For this review, take the finished solid that the model builds, in its own axes (mm). A direction names the side the tool comes from. Coordinates: 2 decimals unless noted, no trailing zeros. Loops run counter-clockwise (first coordinate to the right, second up) from the corner with the lowest first, then second, coordinate; pieces in that order, holes last. Notation, with made-up numbers: (39, -32) - (49, -32) arc R9 cw to (49, -28) - close; hole circle Ø10 at (67.5, -19.5). An arc over 180 degrees is marked (long way). One line per item, written item: value. Start each with the question number.
1. Take a section at C-C, the plane x = 0. Count the separate pieces of the cut face and the enclosed holes in it, and give its area (3 significant figures).
2. To check wall thickness, follow line 1 (X direction, y = 19, z = 0.5); line 2 (X direction, y = 16.75, z = -7); line 3 (Y direction, x = -2.25, z = -12.5). State the ranges of each line that lie inside material, in increasing order. Write a range as from..to.
3. Take a section at B-B, the plane y = 18.25. State the section outline as (x, z) points, and give its area (3 significant figures).
4. Take a section at A-A, the plane x = 3.75. State the section outline as (y, z) points, and give its area (4 significant figures).
5. For faces 1 (the face through (-0.05, 21.48, 1.48)), 2 (the face through (-8, 21, -8)), 3 (the face through (-5, 31, 0)), 4 (the face through (0, 5.98, 3)), list the 3-axis set-ups (+Z, -Z, +X, -X, +Y, -Y) from which the entire face can be reached by the end or side of a thin tool; tool diameter is ignored.
6. The part is to be moulded in two halves that separate along X. For faces 5 (the face through (8.986, 15.805, -12.325)), 6 (the face through (-2.15, 18, 1)), 7 (the face through (10, 22, -6)), say which applies: released by +X, released by -X, zero draft, split by the parting line, or undercut.
7. Insertion check: pin 1 (8 mm diameter, centred on x = 6, z = -17, fed in from +Y); pin 2 (0.9 mm diameter, centred on x = -1.5, y = 6.5, fed in from +Z); pin 3 (6 mm diameter, centred on x = -7.5, y = 23.5, fed in from -Z). Each pin has a flat end and moves straight along its axis. Give the tip position at first contact, or say it passes through.
8. Take a section at D-D, the plane y = 14. State the section outline as (x, z) points.
```python
from build123d import *

# Parameters (mm, degrees)
SKETCH_1_W               = 20
SKETCH_1_H               = 28
EXTRUDE_1_DEPTH          = 3
SKETCH_2_W               = 10
SKETCH_2_H               = 3
CUT_EXTRUDE_1_DEPTH      = 1
SKETCH_3_W               = 4
SKETCH_3_H               = 1
EXTRUDE_2_DEPTH          = 1.5
MIRROR_2_COPY_1_SKETCH_W = 10
MIRROR_2_COPY_1_SKETCH_H = 3
MIRROR_2_COPY_1_DEPTH    = 1
MIRROR_2_COPY_2_SKETCH_W = 4
MIRROR_2_COPY_2_SKETCH_H = 1
MIRROR_2_COPY_2_DEPTH    = 1.5
RIB_2_REACH              = 47.252
SKETCH_4_WALL_W          = 127.859233498
SKETCH_4_WALL_H          = 2


with BuildPart() as part:
    # 草图1 → 凸台-拉伸1 (new body)
    with BuildSketch(Plane.XY):
        with Locations((0, 17.480286539)):
            Rectangle(SKETCH_1_W, SKETCH_1_H)
        with BuildLine():
            Line((2.15, 19.330286539), (2.15, 16.830286539))
            ThreePointArc((2.15, 16.830286539), (0, 14.680286539), (-2.15, 16.830286539))
            Line((-2.15, 16.830286539), (-2.15, 19.330286539))
            ThreePointArc((-2.15, 19.330286539), (0, 21.480286539), (2.15, 19.330286539))
        make_face(mode=Mode.SUBTRACT)
    extrude_1 = extrude(amount=EXTRUDE_1_DEPTH)

    # 草图2 → 切除-拉伸1 (cut)
    with BuildSketch(Plane.XY.offset(3)):
        with Locations((0, 28.480286539)):
            Rectangle(SKETCH_2_W, SKETCH_2_H)
    cut_extrude_1 = extrude(amount=-CUT_EXTRUDE_1_DEPTH, mode=Mode.SUBTRACT)

    # 草图3 → 凸台-拉伸2 (add)
    with BuildSketch(Plane.XY.offset(2)):
        with Locations((0, 29.480286539)):
            Rectangle(SKETCH_3_W, SKETCH_3_H)
    extrude_2 = extrude(amount=EXTRUDE_2_DEPTH)

    # 镜向1: 切除-拉伸1, 凸台-拉伸2 across plane
    add(cut_extrude_1.mirror(Plane.ZX.offset(17.480286539)), mode=Mode.SUBTRACT)
    add(extrude_2.mirror(Plane.ZX.offset(17.480286539)))

    # 镜向2: 凸台-拉伸1, 切除-拉伸1, 凸台-拉伸2 across plane
    add(extrude_1.mirror(Plane(origin=(0, 14.240143269, -14.240143269), x_dir=(0, 0.7071067811865478, 0.7071067811865472), z_dir=(0, -0.7071067811865475, 0.7071067811865477))))
    add(cut_extrude_1.mirror(Plane(origin=(0, 14.240143269, -14.240143269), x_dir=(0, 0.7071067811865478, 0.7071067811865472), z_dir=(0, -0.7071067811865475, 0.7071067811865477))), mode=Mode.SUBTRACT)
    add(extrude_2.mirror(Plane(origin=(0, 14.240143269, -14.240143269), x_dir=(0, 0.7071067811865478, 0.7071067811865472), z_dir=(0, -0.7071067811865475, 0.7071067811865477))))

    # 镜向2 copy 1 sketch → 镜向2 copy 1 (cut)
    with BuildSketch(Plane(origin=(0, 31.480286539, 6.480286539), x_dir=(1, 0, 0), z_dir=(0, 1, 0))):
        with Locations((0, 28.480286539)):
            Rectangle(MIRROR_2_COPY_1_SKETCH_W, MIRROR_2_COPY_1_SKETCH_H)
    extrude(amount=-MIRROR_2_COPY_1_DEPTH, mode=Mode.SUBTRACT)

    # 镜向2 copy 2 sketch → 镜向2 copy 2 (add)
    with BuildSketch(Plane(origin=(0, 30.480286539, 6.480286539), x_dir=(1, 0, 0), z_dir=(0, 1, 0))):
        with Locations((0, 29.480286539)):
            Rectangle(MIRROR_2_COPY_2_SKETCH_W, MIRROR_2_COPY_2_SKETCH_H)
    extrude(amount=MIRROR_2_COPY_2_DEPTH)

    # 草图4 wall → 筋2 (add, up to next)
    with BuildSketch(Plane(origin=(10, 15.980286539, -12.5), x_dir=(0, 0.707106781187, -0.707106781187), z_dir=(0, 0.707106781187, 0.707106781187)), mode=Mode.PRIVATE) as rib_2_sk1:
        with Locations((0, 1)):
            Rectangle(SKETCH_4_WALL_W, SKETCH_4_WALL_H)
    rib_2_tool1 = extrude(rib_2_sk1.sketch, amount=RIB_2_REACH, mode=Mode.PRIVATE) - part.part
    rib_2 = rib_2_tool1.solids().sort_by_distance((10, 15.980286539, -12.5))[0]
    add(rib_2)

    # 镜向3: 筋2 across plane
    add(rib_2.mirror(Plane.ZY))


solid = part.part
```
Solutions:
1. separate pieces: 3
1. enclosed holes: 0
1. area: 113 mm2
2. line 1: -10..-2.15, 2.15..10
2. line 2: -10..-8, 8..10
2. line 3: 28.48..31.48
3. outline: (-10, -14.77) - (-8, -14.77) - (-8, 0) - (-2.15, 0) - (-2.15, 3) - (-10, 3) - close; (2.15, 0) - (8, 0) - (8, -14.77) - (10, -14.77) - (10, 3) - (2.15, 3) - close
3. area: 106 mm2
4. outline: (3.48, 0) - (28.48, 0) - (28.48, -25) - (31.48, -25) - (31.48, -23.5) - (30.48, -23.5) - (30.48, -20.5) - (31.48, -20.5) - (31.48, -1.5) - (30.48, -1.5) - (30.48, 1.5) - (31.48, 1.5) - (31.48, 3) - (28.48, 3) - (28.48, 2) - (26.98, 2) - (26.98, 3) - (7.98, 3) - (7.98, 2) - (4.98, 2) - (4.98, 3) - (3.48, 3) - close
4. area: 148.5 mm2
5. face 1: +Z, -Z
5. face 2: -Z, -Y
5. face 3: +Y
5. face 4: +Z
6. face 5: zero draft
6. face 6: undercut
6. face 7: released by +X
7. pin 1: y = 31.48
7. pin 2: z = 2
7. pin 3: z = -22.98
8. outline: (-10, -10.52) - (-8, -10.52) - (-8, 0) - (8, 0) - (8, -10.52) - (10, -10.52) - (10, 3) - (-10, 3) - close
